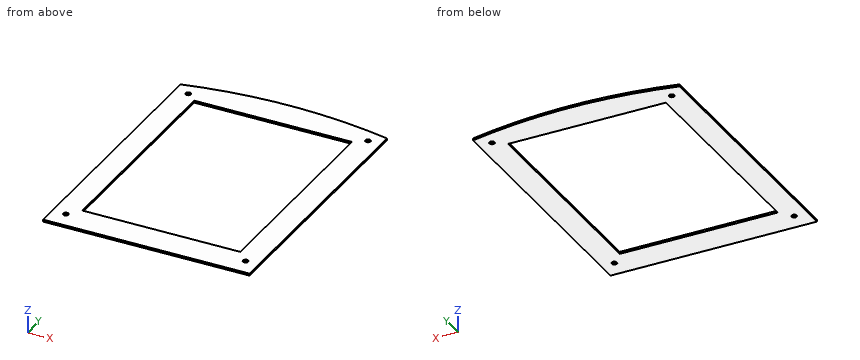
```python
from build123d import *

# Parameters (mm, degrees)
SKETCH1_R           = 2.5
SKETCH1_W           = 153
SKETCH1_H           = 210
BOSS_EXTRUDE1_DEPTH = 2


with BuildPart() as part:
    # Sketch1 → Boss-Extrude1 (new body)
    with BuildSketch(Plane.XY):
        with BuildLine():
            Line((79.989677419, 0), (-120.010322581, 0))
            Line((-120.010322581, 0), (-120.010322581, 258.3))
            add(Edge.make_bspline(
                [(-120.010322581, 258.3), (-22.49451042, 280.450990468), (79.989677419, 258.3)],
                knots=[0, 0, 0, 1, 1, 1], degree=2))
            Line((79.989677419, 258.3), (79.989677419, 0))
        make_face()
        with Locations((-106.803669914, 247.177426871)):
            Circle(SKETCH1_R, mode=Mode.SUBTRACT)
        with Locations((67.322454172, 247.177426871)):
            Circle(SKETCH1_R, mode=Mode.SUBTRACT)
        with Locations((67.322454172, 17.342199543)):
            Circle(SKETCH1_R, mode=Mode.SUBTRACT)
        with Locations((-106.803669914, 17.342199543)):
            Circle(SKETCH1_R, mode=Mode.SUBTRACT)
        with Locations((-20.502905322, 134.178843816)):
            Rectangle(SKETCH1_W, SKETCH1_H, mode=Mode.SUBTRACT)
    extrude(amount=BOSS_EXTRUDE1_DEPTH)


solid = part.part
```
Read the model definition and answer for the solid it produces. Units are mm, in the model's axes. Give positions to 0.01 mm unless a question says otherwise; leave off trailing zeros. Write each loop counter-clockwise with the first axis right and the second up, starting at its lowest first coordinate (ties: lowest second). Pieces come first, ordered by that corner, then holes. Notation, with made-up numbers: M -21.75,67.25 L -5.75,67.25 A34 ccw -5.75,102.25 Z; hole C -30,51 d10. An arc over 180 degrees is marked long. Put each result on its own line as item: value. Start each with the question number.
1. The part is cut by section A-A, the plane y = 81. Give the vertices of the cut face in (x, z), and give its area (3 significant figures).
2. This flat-tipped pin is pushed along its axis until it touches: pin 1 Ø0.6 at (x, z) = (8, 0.5) entering from +Y. Where does it stop, or does it pass through?
3. Consider line 1 along X through (y, z) = (211.5, 0.4); line 2 along Y through (x, z) = (-23, 1.05); line 3 along Y through (x, z) = (40, 0.2). Determine where each line is inside the solid, lowest interval first.
4. The part is cut by section B-B, the plane z = 0.55. Give the number of separate pieces and of enclosed holes in the cut face, and give its area (3 significant figures).
Final values:
1. outline: M -120.01,0 L -97,0 L -97,2 L -120.01,2 Z; M 56,0 L 79.99,0 L 79.99,2 L 56,2 Z
1. area: 94.0 mm²
2. pin 1: stops at y = 268.45
3. line 1: x = -120.01 to -97, 56 to 79.99
3. line 2: y = 0 to 29.18, 239.18 to 269.37
3. line 3: y = 0 to 29.18, 239.18 to 265.28
4. separate pieces: 1
4. enclosed holes: 5
4. area: 20,900 mm²
